Verification items for the finished model (mm, model axes). A direction names the side the tool comes from. Give positions to 0.01 mm unless a question says otherwise; leave off trailing zeros. Write each loop counter-clockwise with the first axis right and the second up, starting at its lowest first coordinate (ties: lowest second). Pieces come first, ordered by that corner, then holes. Notation, with made-up numbers: (1.25, 8.5) -> (12.25, 8.5) arc R9 cw to (12.25, 12.5) -> close; hole circle Ø10 at (7, 26). An arc over 180 degrees is marked (long way). Answer as CSV lines item,"result".
```python
from build123d import *

# Parameters (mm, degrees)
SKETCH1_W           = 50.8
SKETCH1_H           = 533.4
BOSS_EXTRUDE1_DEPTH = 12.7
SKETCH2_W           = 12.7
SKETCH2_H           = 25.4
BOSS_EXTRUDE2_DEPTH = 12.7
SKETCH7_W           = 25.4
SKETCH7_H           = 12.7
CUT_EXTRUDE3_DEPTH  = 538.316573353


with BuildPart() as part:
    # Sketch1 → Boss-Extrude1 (new body)
    with BuildSketch(Plane(origin=(0, 0, 0), x_dir=(1, 0, 0), z_dir=(0, 1, 0))):
        with Locations((25.4, 266.7)):
            Rectangle(SKETCH1_W, SKETCH1_H)
    extrude(amount=BOSS_EXTRUDE1_DEPTH)

    # Sketch2 → Boss-Extrude2 (add, through all)
    with BuildSketch(Plane(origin=(0, 12.7, 0), x_dir=(1, 0, 0), z_dir=(0, 1, 0))):
        with Locations((57.15, 508)):
            Rectangle(SKETCH2_W, SKETCH2_H)
        with Locations((57.15, 447.675)):
            Rectangle(SKETCH2_W, SKETCH2_H)
        with Locations((57.15, 387.35)):
            Rectangle(SKETCH2_W, SKETCH2_H)
        with Locations((57.15, 327.025)):
            Rectangle(SKETCH2_W, SKETCH2_H)
        with Locations((57.15, 266.7)):
            Rectangle(SKETCH2_W, SKETCH2_H)
        with Locations((57.15, 206.375)):
            Rectangle(SKETCH2_W, SKETCH2_H)
        with Locations((57.15, 146.05)):
            Rectangle(SKETCH2_W, SKETCH2_H)
        with Locations((57.15, 85.725)):
            Rectangle(SKETCH2_W, SKETCH2_H)
        with Locations((57.15, 25.4)):
            Rectangle(SKETCH2_W, SKETCH2_H)
    extrude(amount=-BOSS_EXTRUDE2_DEPTH)

    # Sketch7 → Cut-Extrude3 (cut, through all)
    with BuildSketch(Plane(origin=(0, 12.7, 0), x_dir=(1, 0, 0), z_dir=(0, 1, 0))):
        with Locations((25.4, 6.35)):
            Rectangle(SKETCH7_W, SKETCH7_H)
        with Locations((25.4, 527.05)):
            Rectangle(SKETCH7_W, SKETCH7_H)
    extrude(amount=-CUT_EXTRUDE3_DEPTH, mode=Mode.SUBTRACT)


solid = part.part
```
1) Draft check along Z on faces 4 (the flat face through (57, 6, -495.3)), 5 (the flat face through (63.5, 6, -267)). Enter one of: +Z half, -Z half, draft (parallel to the pull), parting line (faces both ways), or undercut.
Reported:
face 4,"undercut"
face 5,"draft"
2) Scan lines: line 1 along Z through (x, y) = (20.5, 0.5); line 2 along X through (y, z) = (4, -356.5). Record each from-to range of solid material in increasing order.
Reported:
line 1,"-520.7 to -12.7"
line 2,"0 to 50.8"
3) Section check A-A (x = 27). Record the boundary of the cut face in (y, z), and give its area (3 significant figures).
Reported:
outline,"(0, -520.7) -> (12.7, -520.7) -> (12.7, -12.7) -> (0, -12.7) -> close"
area,"6,450 mm²"
4) Tool access check on faces 1 (the flat face through (57, 6, -314.325)), 2 (the flat face through (12.7, 6, -527)), 3 (the flat face through (63.5, 6, -387)). Record the directions out of +Z, -Z, +X, -X, +Y, -Y that give a thin tool (end or side, any length) a straight path to the whole face; none if there is none.
Reported:
face 1,"+X, +Y, -Y"
face 2,"-Z, +Y, -Y"
face 3,"+Z, -Z, +X, +Y, -Y"
5) Section check B-B (z = -57). Record the boundary of the cut face in (x, y).
Reported:
outline,"(0, 0) -> (50.8, 0) -> (50.8, 12.7) -> (0, 12.7) -> close"
6) Depth check by flat-ended pin: pin 1 (2 mm diameter, centred on x = 28, y = 7, fed in from -Z); pin 2 (4 mm diameter, centred on x = 55, y = 6.5, fed in from +Z); pin 3 (1.5 mm diameter, centred on y = 3, z = -68, fed in from +X). Enter the tip coordinate at first touch or a pass-through.
Reported:
pin 1,"z = -520.7"
pin 2,"z = -12.7"
pin 3,"x = 50.8"
